from build123d import *

# Parameters (mm, degrees)
SKETCH_3_W             = 0.64
SKETCH_3_H             = 0.64
CHAMFER_1_SIZE         = 0.15
CHAMFER_1_SIZE2        = 0.259807621
CHAMFER_1_PART_2_SIZE  = 0.15
CHAMFER_1_PART_2_SIZE2 = 0.259807621
SKETCH1_W              = 0.64
SKETCH1_H              = 4.734584987
CUT_EXTRUDE1_DEPTH     = 8.57


with BuildPart() as part:
    # Sweep 1: sweep along a path in Sketch 2
    with BuildLine(Plane(origin=(0, 0, 0), x_dir=(0, 0, -1), z_dir=(1, 0, 0))) as sweep_1_path:
        Line((0, -3), (0, 0))
        Line((0, 0), (0, 4.75))
        ThreePointArc((0, 4.75), (0.292893219, 5.457106781), (1, 5.75))
        Line((1, 5.75), (7.25, 5.75))
    # Sketch 3 → Sweep 1 (sweep)
    with BuildSketch(Plane(origin=(0, 0, 0), x_dir=(1, 0, 0), z_dir=(0, 1, 0))):
        Rectangle(SKETCH_3_W, SKETCH_3_H)
    sweep(path=sweep_1_path.line)

    # Chamfer 1
    chamfer_1_edges = [part.edges().sort_by_distance(p)[0] for p in [
        (0, 5.43, -7.25),
        (-0.32, 5.75, -7.25),
        (0, 6.07, -7.25),
        (0.32, 5.75, -7.25),
    ]]
    chamfer_1_side = [part.faces().sort_by_distance(p)[0] for p in [
        (0, 5.75, -7.25),
    ]]
    chamfer(chamfer_1_edges, length=CHAMFER_1_SIZE, length2=CHAMFER_1_SIZE2, reference=chamfer_1_side[0])

    # Chamfer 1 part 2
    chamfer_1_part_2_edges = [part.edges().sort_by_distance(p)[0] for p in [
        (0.32, -3, 0),
        (0, -3, -0.32),
        (-0.32, -3, 0),
        (0, -3, 0.32),
    ]]
    chamfer_1_part_2_side = [part.faces().sort_by_distance(p)[0] for p in [
        (0, -3, 0),
    ]]
    chamfer(chamfer_1_part_2_edges, length=CHAMFER_1_PART_2_SIZE, length2=CHAMFER_1_PART_2_SIZE2, reference=chamfer_1_part_2_side[0])

    # Sketch1 → Cut-Extrude1 (cut, through all)
    with BuildSketch(Plane.XY.offset(0.32)):
        with Locations((0, -0.874507109)):
            Rectangle(SKETCH1_W, SKETCH1_H)
    extrude(amount=-CUT_EXTRUDE1_DEPTH, mode=Mode.SUBTRACT)


solid = part.part
Source: CAD feature listing. Evaluate the final solid. Frame: model axes, mm. Round coordinates to 2 decimals unless told otherwise and drop trailing zeros. Loops run counter-clockwise (first coordinate to the right, second up) from the corner with the lowest first, then second, coordinate; pieces in that order, holes last. Notation, with made-up numbers: (-17, 60.5) - (11, 60.5) arc R11 ccw to (11, 71.5) - close; hole circle Ø1 at (37, -3.75). An arc over 180 degrees is marked (long way). Write item = value, one per line. Start each with the question number.
Item 1: Material intervals for line 1 (Z direction, x = 0.2, y = 3.1); line 2 (Y direction, x = 0.15, z = -5.5); line 3 (Z direction, x = 0, y = 5.65), sorted ascending.
Item 2: Section query B-B on y = 4.4. Output: boundary loops of the cut face in (x, z), plus the area to 3 significant figures.
Item 3: Section query A-A on x = 0.05. Output: boundary loops of the cut face in (y, z), plus the area to 3 significant figures.
Item 4: Section query C-C on z = -4. Output: boundary loops of the cut face in (x, y), plus the area to 3 significant figures.
Results list:
q1.line_1 = -0.32 to 0.32
q1.line_2 = 5.43 to 6.07
q1.line_3 = -7.25 to -0.03
q2.outline = (-0.32, -0.32) - (0.32, -0.32) - (0.32, 0.32) - (-0.32, 0.32) - close
q2.area = 0.410 mm²
q3.outline = (1.49, -0.32) - (4.75, -0.32) arc R0.68 cw to (5.43, -1) - (5.43, -6.99) - (5.58, -7.25) - (5.92, -7.25) - (6.07, -6.99) - (6.07, -1) arc R1.32 ccw to (4.75, 0.32) - (1.49, 0.32) - close
q3.area = 7.05 mm²
q4.outline = (-0.32, 5.43) - (0.32, 5.43) - (0.32, 6.07) - (-0.32, 6.07) - close
q4.area = 0.410 mm²
